Here's the drawing with two shaded views (mm, measured from the low corner). I have some questions. Give positions to 0.01 mm unless a question says otherwise; leave off trailing zeros. Write each loop counter-clockwise with the first axis right and the second up, starting at its lowest first coordinate (ties: lowest second). Pieces come first, ordered by that corner, then holes. Notation, with made-up numbers: (46, 21) - (94, 21) arc R27 cw to (94, 48) - close; hole circle Ø4 at (28.5, -5.75). An arc over 180 degrees is marked (long way). Write item = value, one per line.
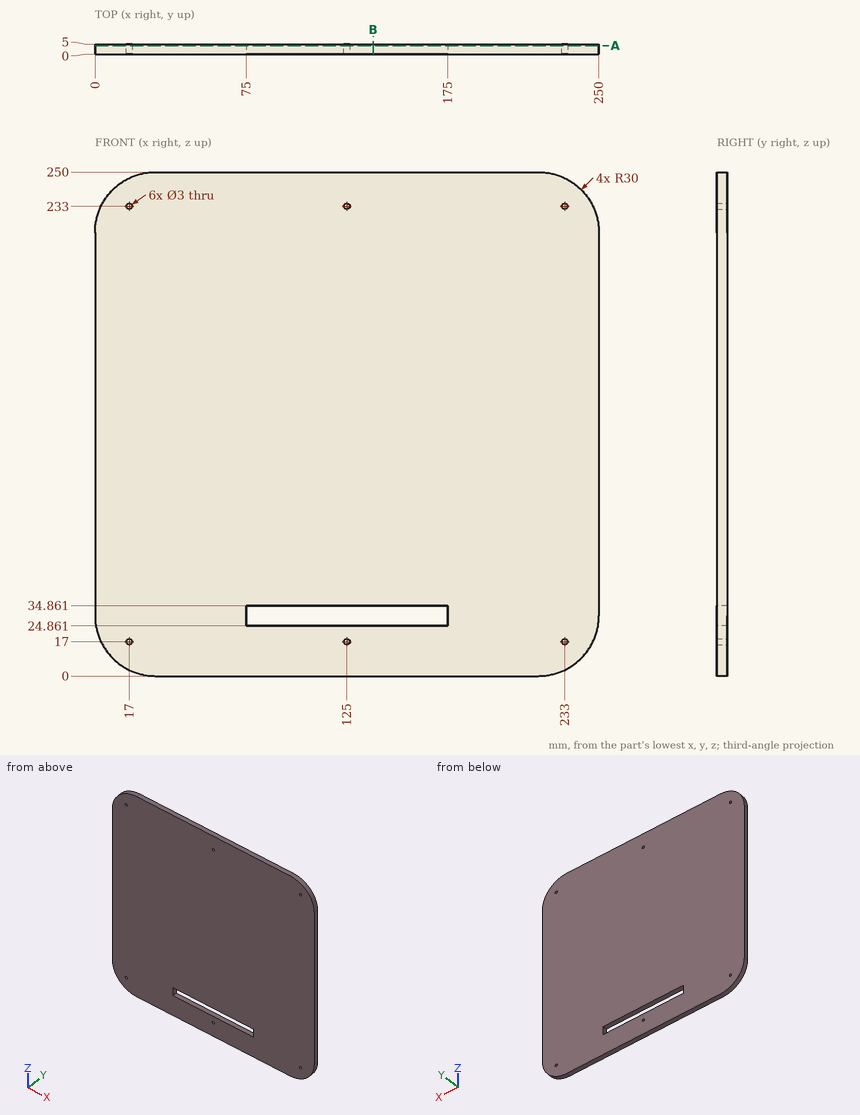
1. If we section it at B-B, the plane x = 138: Please give me the cut outline in (y, z), and give its area (3 significant figures).
Filled sheet:
outline = (0, 0) - (5, 0) - (5, 24.86) - (0, 24.86) - close; (0, 34.86) - (5, 34.86) - (5, 250) - (0, 250) - close
area = 1,200 mm2
2. If we section it at A-A, the plane y = 4.2: Please give me the cut outline in (x, z).
Filled sheet:
outline = (0, 30) arc R30 ccw to (30, 0) - (220, 0) arc R30 ccw to (250, 30) - (250, 220) arc R30 ccw to (220, 250) - (30, 250) arc R30 ccw to (0, 220) - close; hole circle Ø3 at (17, 17); hole circle Ø3 at (17, 233); hole (75, 24.86) - (175, 24.86) - (175, 34.86) - (75, 34.86) - close; hole circle Ø3 at (125, 17); hole circle Ø3 at (125, 233); hole circle Ø3 at (233, 17); hole circle Ø3 at (233, 233)
3. I need wall thicknesses on line 1 (Z direction, x = 125, y = 2.5); line 2 (Z direction, x = 17.5, y = 4.6); line 3 (X direction, y = 1.8, z = 17). Which ranges of each line are inside material? Lowest first, please.
Filled sheet:
line_1 = 0 to 15.5, 18.5 to 24.86, 34.86 to 231.5, 234.5 to 250
line_2 = 2.73 to 15.59, 18.41 to 231.59, 234.41 to 247.27
line_3 = 2.96 to 15.5, 18.5 to 123.5, 126.5 to 231.5, 234.5 to 247.04
